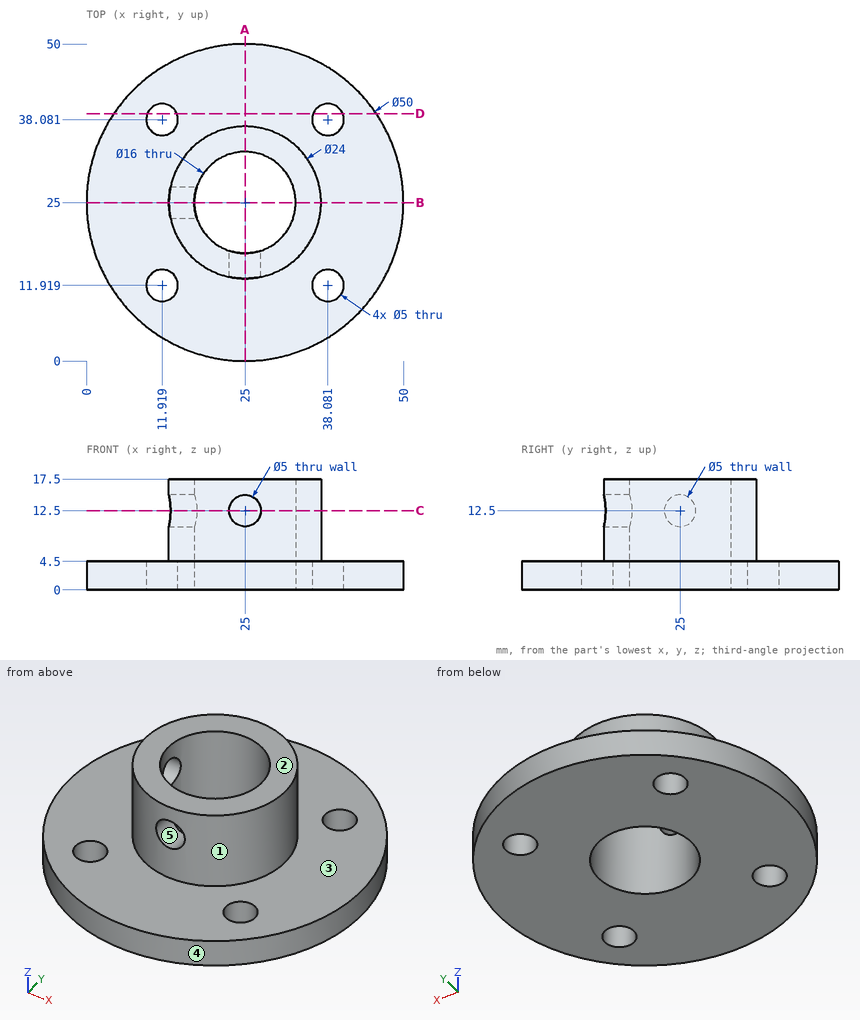
Source: three-view drawing plus pictorial views. Frame: mm from the lowest corner of the part. A direction names the side the tool comes from. Round coordinates to 2 decimals unless told otherwise and drop trailing zeros. Loops run counter-clockwise (first coordinate to the right, second up) from the corner with the lowest first, then second, coordinate; pieces in that order, holes last.
1. Ray query, L1, parallel to Z at x = 25, y = 14.85; L2, parallel to X at y = 25, z = 6.25; L3, parallel to Z at x = 35.5, y = 3.5. Return the intervals inside material, ascending.
2. Access query for the marked faces 1 and 2. Directions: +Z, -Z, +X, -X, +Y, -Y. A direction counts if a zero-diameter tool reaches every point of the face in a straight line with its end or side. Return the directions, or none.
3. Mould query, pull axis X, two halves, no side actions, for the marked faces 3, 4 and 5. Classes: released by +X, released by -X, zero draft, split by the parting line, or undercut.
4. Section query D-D on y = 39. Output: boundary loops of the cut face in (x, z).
5. Contact query for flat-ended pins moving along their axis: pin 1 (4.5 mm diameter, centred on y = 25, z = 12.5, fed in from +X); pin 2 (6 mm diameter, centred on x = 8.5, z = 4.5, fed in from -Y); pin 3 (6 mm diameter, centred on x = 38.08, y = 38.08, fed in from +Z). Output: stop coordinate, or through.
6. Section query A-A on x = 25. Output: boundary loops of the cut face in (y, z), and give its area (3 significant figures).
7. Section query C-C on z = 12.5. Output: boundary loops of the cut face in (x, y), and give its area (3 significant figures).
Answers below:
1. L1: z = 0 to 10, 15 to 17.5
1. L2: x = 13 to 17, 33 to 37
1. L3: z = 0 to 4.5
2. face 1: +Z
2. face 2: +Z, +X, -X, +Y, -Y
3. face 3: zero draft
3. face 4: split by the parting line
3. face 5: undercut
4. outline: (4.29, 0) - (9.59, 0) - (9.59, 4.5) - (4.29, 4.5) - close; (14.24, 0) - (35.76, 0) - (35.76, 4.5) - (14.24, 4.5) - close; (40.41, 0) - (45.71, 0) - (45.71, 4.5) - (40.41, 4.5) - close
5. pin 1: stops at x = 37
5. pin 2: stops at y = 3.96
5. pin 3: stops at z = 4.5
6. outline: (0, 0) - (17, 0) - (17, 10) - (13, 10) - (13, 4.5) - (0, 4.5) - close; (13, 15) - (17, 15) - (17, 17.5) - (13, 17.5) - close; (33, 0) - (50, 0) - (50, 4.5) - (37, 4.5) - (37, 17.5) - (33, 17.5) - close
6. area: 237 mm2
7. outline: (13.26, 22.5) arc R12 ccw to (22.5, 13.26) - (22.5, 17.4) arc R8 cw to (17.4, 22.5) - close; (13.26, 27.5) - (17.4, 27.5) arc R8 cw (long way) to (27.5, 17.4) - (27.5, 13.26) arc R12 ccw (long way) to start
7. area: 211 mm2
